Study the drawing (mm; zero at the part's minimum x, y, z) and answer. A direction names the side the tool comes from. Give positions to 0.01 mm unless a question says otherwise; leave off trailing zeros. Order: outer loops, then holes, each group sorted by start corner. A loop starts at its lowest first (then second) coordinate and runs counter-clockwise, first axis right, second up.
Item 1: A cutting plane is placed at A-A (y = 6.75). Write down the section's boundary in (x, z), plus the area to 3 significant figures.
Item 2: A cutting plane is placed at D-D (x = 10). Write down the section's boundary in (y, z).
Item 3: A cutting plane is placed at C-C (z = 10.75). Write down the section's boundary in (x, y).
Item 4: Find the intervals of material crossed by line 1 along Y through (x, z) = (17, 5.5); line 2 along X through (y, z) = (1.5, 10.8); line 3 along X through (y, z) = (5.5, 11), in increasing order.
Item 5: Which of the six approach directions +Z, -Z, +X, -X, +Y, -Y give full straight-line access (tool end or side, diameter ignored) to the marked faces 4 and 5?
Item 6: A cutting plane is placed at B-B (x = 7). Write down the section's boundary in (y, z).
Item 7: Given pin 1 Ø1.6 at (x, z) = (10, 1.2) entering from +Y, flat-ended and moving along its own axis, determine where the tip first touches the part or whether it passes through.
Item 8: The mould has two halves that part along X. Classify the marked faces 1, 2 and 3: +X half, -X half, draft (parallel to the pull), parting line (faces both ways), or undercut.
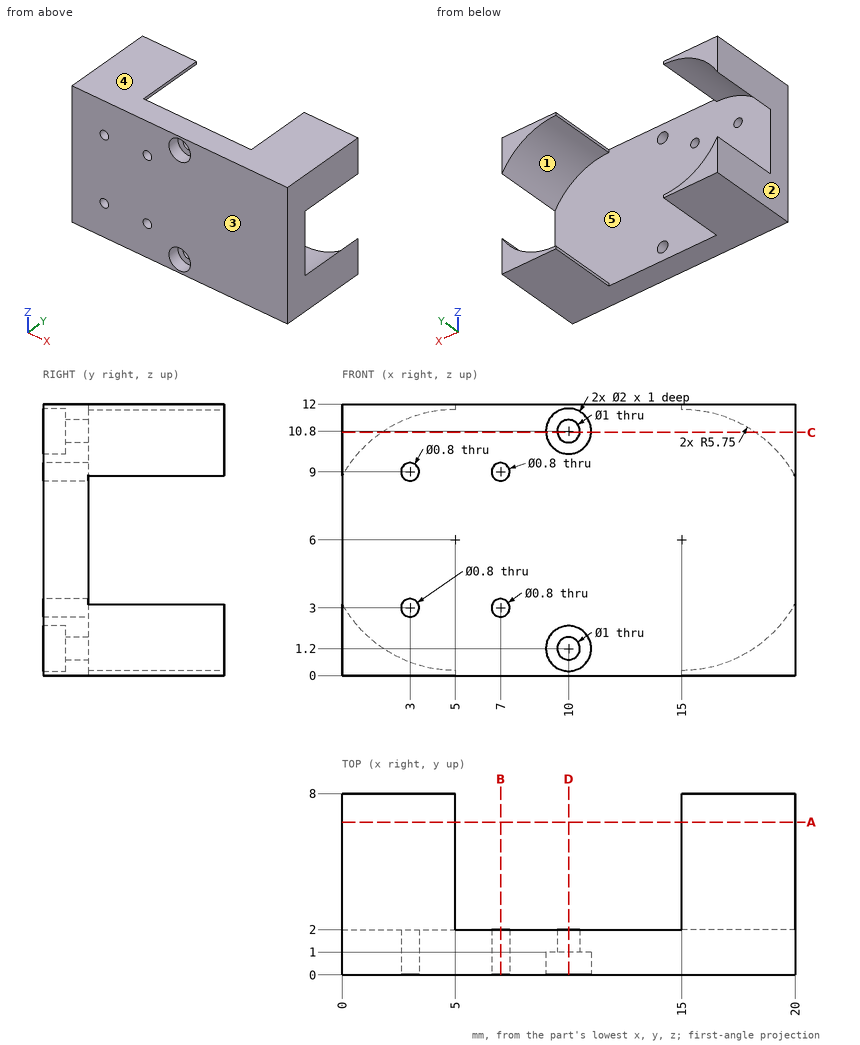
Response values:
1. outline: (0, 0) - (5, 0) - (5, 0.25) arc R5.75 cw to (0, 3.16) - close; (0, 8.84) arc R5.75 cw to (5, 11.75) - (5, 12) - (0, 12) - close; (15, 0) - (20, 0) - (20, 3.16) arc R5.75 cw to (15, 0.25) - close; (15, 11.75) arc R5.75 cw to (20, 8.84) - (20, 12) - (15, 12) - close
1. area: 21.9 mm2
2. outline: (0, 0) - (2, 0) - (2, 0.7) - (1, 0.7) - (1, 0.2) - (0, 0.2) - close; (0, 2.2) - (1, 2.2) - (1, 1.7) - (2, 1.7) - (2, 10.3) - (1, 10.3) - (1, 9.8) - (0, 9.8) - close; (0, 11.8) - (1, 11.8) - (1, 11.3) - (2, 11.3) - (2, 12) - (0, 12) - close
3. outline: (0, 0) - (9, 0) - (9, 1) - (9.5, 1) - (9.5, 2) - (1.76, 2) - (1.76, 8) - (0, 8) - close; (10.5, 1) - (11, 1) - (11, 0) - (20, 0) - (20, 8) - (18.24, 8) - (18.24, 2) - (10.5, 2) - close
4. line 1: y = 0 to 2
4. line 2: x = 0 to 9.5, 10.5 to 20
4. line 3: x = 0 to 2.16, 17.84 to 20
5. face 4: +Z, +X, -X, +Y, -Y
5. face 5: +Y
6. outline: (0, 0) - (2, 0) - (2, 2.6) - (0, 2.6) - close; (0, 3.4) - (2, 3.4) - (2, 8.6) - (0, 8.6) - close; (0, 9.4) - (2, 9.4) - (2, 12) - (0, 12) - close
7. pin 1: stops at y = 2
8. face 1: undercut
8. face 2: -X half
8. face 3: draft
